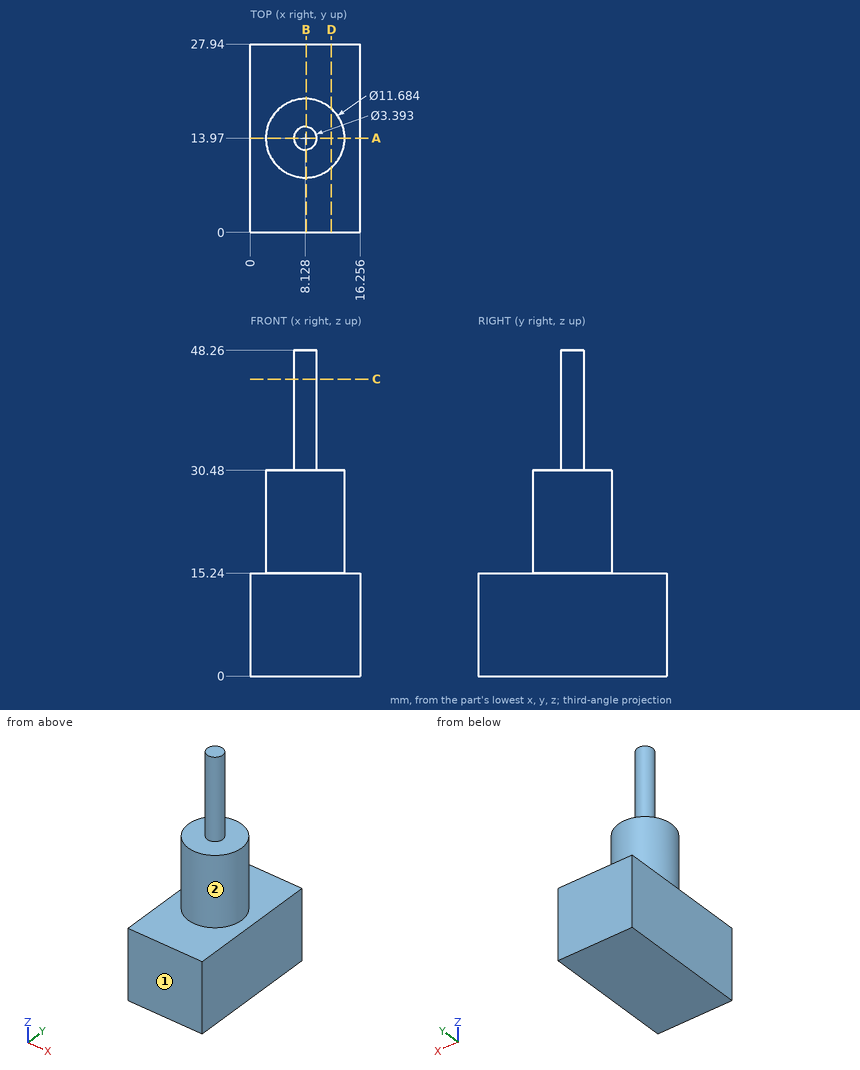
For this review, use the dimensioned drawing (mm, ordinates from the lowest corner) and the shaded views. A direction names the side the tool comes from. Coordinates: 2 decimals unless noted, no trailing zeros. Loops run counter-clockwise (first coordinate to the right, second up) from the corner with the lowest first, then second, coordinate; pieces in that order, holes last. Notation, with made-up numbers: (74, -39.5) -> (107, -39.5) arc R12 ccw to (107, -17.5) -> close; hole circle Ø6 at (-1.75, -1). An arc over 180 degrees is marked (long way). Return JSON: item names as keys, results as strings. Group by question number.
(1) Tool access review of the marked faces 1 and 2: name each direction out of +Z, -Z, +X, -X, +Y, -Y from which nothing blocks a thin tool from reaching the whole face with its end or side.
(2) Consider section B-B, the plane x = 8.25. Give the boundary of the cut face in (y, z), plus the area to 3 significant figures.
(3) For pin 1 Ø8 at (x, y) = (11, 19.5) entering from +Z; pin 2 Ø1.5 at (y, z) = (19.5, 28) entering from -X; pin 3 Ø4 at (y, z) = (14.5, 35) entering from +X (1 decimal); pin 4 Ø10 at (y, z) = (18, 13.5) entering from -X, all flat-tipped, find the tip position at first contact; note any pin that passes through.
(4) Consider section A-A, the plane y = 13.97. Give the boundary of the cut face in (x, z) (1 decimal), plus the area to 3 significant figures.
(5) Consider section D-D, the plane x = 12. Give the boundary of the cut face in (y, z) (1 decimal).
(6) To check wall thickness, follow L1, parallel to Z at x = 5.5, y = 12.5; L2, parallel to Z at x = 10, y = 1.5; L3, parallel to Y at x = 9.5, z = 25. State the ranges of each line that lie inside material, in increasing order.
(7) Consider section C-C, the plane z = 44. Give the boundary of the cut face in (x, y) (1 decimal).
Results below:
{
 "1": {"face 1": "+Z, -Z, +X, -X, -Y", "face 2": "+Z"},
 "2": {"outline": "(0, 0) -> (27.94, 0) -> (27.94, 15.24) -> (19.81, 15.24) -> (19.81, 30.48) -> (15.66, 30.48) -> (15.66, 48.26) -> (12.28, 48.26) -> (12.28, 30.48) -> (8.13, 30.48) -> (8.13, 15.24) -> (0, 15.24) -> close", "area": "664 mm2"},
 "3": {"pin 1": "stops at z = 30.48", "pin 2": "stops at x = 4.77", "pin 3": "stops at x = 9.8", "pin 4": "stops at x = 0"},
 "4": {"outline": "(0, 0) -> (16.3, 0) -> (16.3, 15.2) -> (14, 15.2) -> (14, 30.5) -> (9.8, 30.5) -> (9.8, 48.3) -> (6.4, 48.3) -> (6.4, 30.5) -> (2.3, 30.5) -> (2.3, 15.2) -> (0, 15.2) -> close", "area": "486 mm2"},
 "5": {"outline": "(0, 0) -> (27.9, 0) -> (27.9, 15.2) -> (18.3, 15.2) -> (18.3, 30.5) -> (9.6, 30.5) -> (9.6, 15.2) -> (0, 15.2) -> close"},
 "6": {"L1": "z = 0 to 30.48", "L2": "z = 0 to 15.24", "L3": "y = 8.29 to 19.65"},
 "7": {"outline": "circle Ø3.4 at (8.1, 14)"}
}
